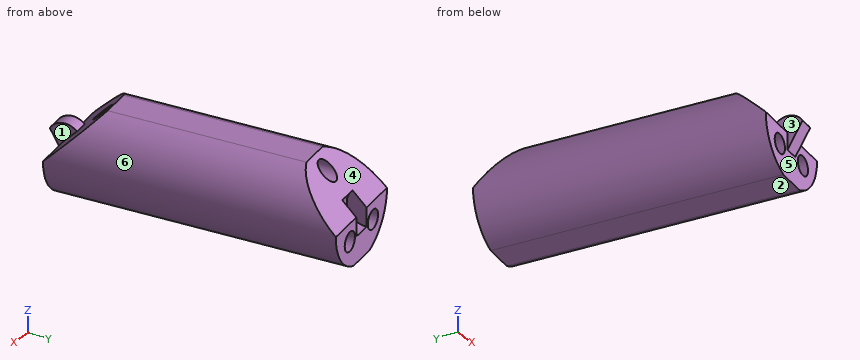
```python
from build123d import *

# Parameters (mm, degrees)
SKETCH3_R               = 8
BOSS_EXTRUDE1_DEPTH     = 47.368421053
CUT_EXTRUDE1_DEPTH      = 13.860013886
CUT_EXTRUDE1_DEPTH_BACK = 13.860013886
BOSS_EXTRUDE2_DEPTH     = 1.2
CUT_EXTRUDE2_DEPTH      = 1.6
SKETCH8_R               = 1.4
SKETCH8_R_2             = 1.6
CUT_EXTRUDE3_DEPTH      = 2.64160469
CUT_EXTRUDE3_DEPTH_BACK = 51.711414178
CUT_EXTRUDE4_DEPTH      = 51.711414178


with BuildPart() as part:
    # Sketch3 → Boss-Extrude1 (new body)
    with BuildSketch(Plane(origin=(-20.344467381, 196.178792599, 0), x_dir=(-0.994665758, -0.103150523, 0), z_dir=(0.103150523, -0.994665758, 0))):
        with Locations((-10.431405186, 0)):
            Circle(SKETCH3_R)
    extrude(amount=BOSS_EXTRUDE1_DEPTH)

    # Sketch4 → Cut-Extrude1 (cut, two sides)
    with BuildSketch(Plane(origin=(10.375761543, 1.076004901, 0), x_dir=(0.103150523, -0.994665758, 0), z_dir=(-0.994665758, -0.103150523, 0))) as cut_extrude1_sk:
        Polygon((-197.230869842, 0), (-189.230869842, 8), (-197.230869842, 8), align=None)
        Polygon((-157.862448789, 8), (-149.862448789, 8), (-149.862448789, 0), align=None)
    extrude(amount=CUT_EXTRUDE1_DEPTH, mode=Mode.SUBTRACT)
    extrude(cut_extrude1_sk.sketch, amount=-CUT_EXTRUDE1_DEPTH_BACK, mode=Mode.SUBTRACT)

    # Sketch5 → Boss-Extrude2 (add, symmetric)
    with BuildSketch(Plane(origin=(10.375761543, 1.076004901, 0), x_dir=(0.103150523, -0.994665758, 0), z_dir=(-0.994665758, -0.103150523, 0))):
        with BuildLine():
            Line((-149.862448789, -2.8), (-147.437577659, 1.4))
            ThreePointArc((-147.437577659, 1.4), (-149.496975451, 2.776045612), (-151.842347777, 1.979898987))
            Line((-151.842347777, 1.979898987), (-149.862448789, 0))
            Line((-149.862448789, 0), (-149.862448789, -2.8))
        make_face()
    extrude(amount=BOSS_EXTRUDE2_DEPTH, both=True)

    # Sketch7 → Cut-Extrude2 (cut, symmetric)
    with BuildSketch(Plane(origin=(10.375761543, 1.076004901, 0), x_dir=(0.103150523, -0.994665758, 0), z_dir=(-0.994665758, -0.103150523, 0))):
        with BuildLine():
            Line((-194.968128142, 2.2627417), (-197.230869842, 0))
            Line((-197.230869842, 0), (-197.230869842, -3.2))
            ThreePointArc((-197.230869842, -3.2), (-194.274455338, -1.224586984), (-194.968128142, 2.2627417))
        make_face()
    extrude(amount=CUT_EXTRUDE2_DEPTH, both=True, mode=Mode.SUBTRACT)

    # Sketch8 → Cut-Extrude3 (cut, two sides)
    with BuildSketch(Plane(origin=(-20.344467381, 196.178792599, 0), x_dir=(0.994665758, 0.103150523, 0), z_dir=(-0.103150523, 0.994665758, 0))) as cut_extrude3_sk:
        with Locations((10.431405186, -5.5)):
            Circle(SKETCH8_R)
        with Locations((6.831405186, 3)):
            Circle(SKETCH8_R_2)
        with Locations((14.031405186, 3)):
            Circle(SKETCH8_R_2)
    extrude(amount=CUT_EXTRUDE3_DEPTH, mode=Mode.SUBTRACT)
    extrude(cut_extrude3_sk.sketch, amount=-CUT_EXTRUDE3_DEPTH_BACK, mode=Mode.SUBTRACT)

    # Sketch9 → Cut-Extrude4 (cut, through all)
    with BuildSketch(Plane(origin=(-20.344467381, 196.178792599, 0), x_dir=(0.994665758, 0.103150523, 0), z_dir=(-0.103150523, 0.994665758, 0))):
        with BuildLine():
            Line((7.933405986, 7.6), (12.929404385, 7.6))
            ThreePointArc((12.929404385, 7.6), (10.431405186, 8), (7.933405986, 7.6))
        make_face()
        with BuildLine():
            Line((7.933405986, -7.6), (12.929404385, -7.6))
            ThreePointArc((12.929404385, -7.6), (10.431405186, -8), (7.933405986, -7.6))
        make_face()
    extrude(amount=-CUT_EXTRUDE4_DEPTH, mode=Mode.SUBTRACT)


solid = part.part
```
Here's how the part is built. I have some questions about the finished solid (model axes, mm). Face numbers are marked on the shaded views. A direction names the side the tool comes from. Coordinates: 2 decimals unless noted, no trailing zeros. Write each loop counter-clockwise with the first axis right and the second up, starting at its lowest first coordinate (ties: lowest second). Pieces come first, ordered by that corner, then holes. Notation, with made-up numbers: (54.25, 0) -> (72.25, 0) arc R33 ccw to (72.25, 31) -> close; hole circle Ø2 at (56, -25). An arc over 180 degrees is marked (long way). Use a Markdown table: item, result. Add a question column.
(1) Please list where these lines run through material, in increasing order: line 1 (X direction, y = 183, z = -2.25); line 2 (X direction, y = 171.5, z = 5); line 3 (X direction, y = 190, z = -4).
(2) If we section it at A-A, the plane z = 0.5: Write out the boundary of the cut face in (x, y).
(3) I'm going to push flat-ended pins straight in: P1, Ø1.5, axis at y = 174, z = 4, coming from the +X side; P2, Ø3, axis at y = 159, z = 1, coming from the -X side; P3, Ø1, axis at x = -2.5, y = 193, coming from the +Z side; P4, Ø12, axis at x = -13, y = 174.5, coming from the -Z side. Where does each tip first touch, or does it pass through?
(4) We'd pull the mould along X, two halves only. Please class the marked faces 3, 4, 5 and 6: +X half, -X half, draft (parallel to the pull), parting line (faces both ways), or undercut.
(5) If we section it at B-B, the plane y = 164: State how many separate pieces and enclosed holes the cut face has, and give its area (3 significant figures).
(6) For the marked faces 1 and 2, which set-ups out of +Z, -Z, +X, -X, +Y, -Y let a thin tool reach every point of the face, with its end or its side?
Outcome:
| question | item | result |
|---|---|---|
| 1 | line 1 | x = -16.21 to -13.53, -10.69 to -6.29, -3.45 to -0.77 |
| 1 | line 2 | x = -13.58 to -8.61, -5.98 to -1.02 |
| 1 | line 3 | x = -16.18 to -14.09, -11.58 to -6.85, -4.34 to -2.25 |
| 2 | outline | (-17.86, 195.93) -> (-13.08, 149.81) -> (-6.33, 150.51) -> (-6.08, 148.12) -> (-3.69, 148.37) -> (-3.94, 150.76) -> (2.81, 151.46) -> (-1.98, 197.58) -> (-8.33, 196.92) -> (-8.05, 194.28) -> (-11.23, 193.95) -> (-11.51, 196.59) -> close |
| 3 | P1 | stops at x = -0.2 |
| 3 | P2 | stops at x = -14.18 |
| 3 | P3 | stops at z = 4.68 |
| 3 | P4 | stops at z = -7.6 |
| 4 | face 3 | undercut |
| 4 | face 4 | -X half |
| 4 | face 5 | undercut |
| 4 | face 6 | +X half |
| 5 | separate pieces | 1 |
| 5 | enclosed holes | 3 |
| 5 | area | 177 mm^2 |
| 6 | face 1 | +Z, +X |
| 6 | face 2 | -Z, +X, -X, +Y, -Y |
